Verification items for the finished model (mm, model axes). A direction names the side the tool comes from. Round coordinates to 2 decimals unless told otherwise and drop trailing zeros. Loops run counter-clockwise (first coordinate to the right, second up) from the corner with the lowest first, then second, coordinate; pieces in that order, holes last.
from build123d import *

# Parameters (mm, degrees)
EXTRUDE_1_DEPTH     = 90
CUT_EXTRUDE_1_DEPTH = 160
SKETCH_4_W          = 100
SKETCH_4_H          = 40
CUT_EXTRUDE_2_DEPTH = 102.056914657
SKETCH_5_R          = 5
CUT_EXTRUDE_3_DEPTH = 102.056914657
SKETCH_6_R          = 2.5
CUT_EXTRUDE_4_DEPTH = 102.056914657


with BuildPart() as part:
    # 草圖1 → 填料-伸長1 (new, symmetric)
    with BuildSketch(Plane(origin=(0, 0, 0), x_dir=(0, 0, -1), z_dir=(1, 0, 0))):
        Polygon((-59.343145751, 0), (-13.343145751, 46), (0, 46), (0, 50), (-15, 50), (-62.171572875, 2.828427125), align=None)
    extrude(amount=EXTRUDE_1_DEPTH, both=True)

    # 草圖3 → 除料-伸長1 (cut)
    with BuildSketch(Plane(origin=(0, 0, 0), x_dir=(1, 0, 0), z_dir=(0, 1, 0))):
        Polygon((-90, -15), (-90, -62.171572875), (-80, -62.171572875), align=None)
        Polygon((90, -15), (80, -62.171572875), (90, -62.171572875), align=None)
    extrude(amount=CUT_EXTRUDE_1_DEPTH, mode=Mode.SUBTRACT)

    # 草圖4 → 除料-伸長2 (cut, through all)
    with BuildSketch(Plane(origin=(0, 32.5, 32.5), x_dir=(1, 0, 0), z_dir=(0, 0.7071067811865467, 0.7071067811865485))):
        with Locations((-15, -11.961940777)):
            Rectangle(SKETCH_4_W, SKETCH_4_H)
    extrude(amount=-CUT_EXTRUDE_2_DEPTH, mode=Mode.SUBTRACT)

    # 草圖5 → 除料-伸長3 (cut, through all)
    with BuildSketch(Plane(origin=(0, 32.5, 32.5), x_dir=(1, 0, 0), z_dir=(0, 0.7071067811865467, 0.7071067811865485))):
        with Locations(Location((60, -11.961940777, 0), (0, 0, 270))):
            Circle(SKETCH_5_R)
    extrude(amount=-CUT_EXTRUDE_3_DEPTH, mode=Mode.SUBTRACT)

    # 草圖6 → 除料-伸長4 (cut, through all)
    with BuildSketch(Plane(origin=(0, 32.5, 32.5), x_dir=(1, 0, 0), z_dir=(0, 0.7071067811865467, 0.7071067811865485))):
        with Locations(Location((70, -31.961940777, 0), (0, 0, 270))):
            Circle(SKETCH_6_R)
        with Locations(Location((70, 18.038059223, 0), (0, 0, 270))):
            Circle(SKETCH_6_R)
    cut_extrude_4 = extrude(amount=-CUT_EXTRUDE_4_DEPTH, mode=Mode.SUBTRACT)

    # 鏡射1: 除料-伸長4 across plane
    add(cut_extrude_4.mirror(Plane(origin=(0, 0, 0), x_dir=(0, 0, 1), z_dir=(1, 0, 0))), mode=Mode.SUBTRACT)


solid = part.part
1. Section check A-A (x = -27). Enter the section's corners in (y, z), then the cut area to 3 significant figures.
2. Gauge pin test, flat ends, axial feed: P1, Ø15.5, axis at y = 25.5, z = 34, coming from the +X side; P2, Ø3, axis at y = 42, z = 22, coming from the -X side; P3, Ø6.5, axis at x = 5.5, z = 5, coming from the -Y side. Record the tip position at first contact, or that the pin passes through.
3. Section check D-D (x = 40). Enter the section's corners in (y, z).
4. Section check B-B (y = 14.5). Enter the section's corners in (x, z).
5. Release check for a two-part mould opening along X. For faces 1 (the face through (-84.977, 24.883, 38.696)), 2 (the face through (67.56, 44.24, 17.97)), 3 (the face through (1, 50, 7)), 4 (the face through (85.023, 24.883, 38.476)) record: released by +X, released by -X, zero draft, split by the parting line, or undercut.
6. Scan lines: L1, parallel to X at y = 9, z = 53; L2, parallel to Y at x = -61.5, z = 12; L3, parallel to X at y = 3, z = 59.5. Record each from-to range of solid material in increasing order.
7. Section check C-C (z = 48). Enter the section's corners in (x, y), then the cut area to 3 significant figures.
8. Tool access check on faces 5 (the face through (1, 48, 0)), 6 (the face through (1, 46, 7)). Record the directions out of +Z, -Z, +X, -X, +Y, -Y that give a thin tool (end or side, any length) a straight path to the whole face; none if there is none.
Taken from the geometry:
1. outline: (0, 59.34) - (7.07, 52.27) - (9.9, 55.1) - (2.83, 62.17) - close; (35.36, 23.99) - (46, 13.34) - (46, 0) - (50, 0) - (50, 15) - (38.18, 26.82) - close
1. area: 160 mm2
2. P1: stops at x = 87.15
2. P2: stops at x = -88.83
2. P3: stops at y = 46
3. outline: (0, 59.34) - (46, 13.34) - (46, 0) - (50, 0) - (50, 15) - (2.83, 62.17) - close
4. outline: (-83.67, 44.84) - (-65, 44.84) - (-65, 50.5) - (-82.47, 50.5) - close; (35, 44.84) - (83.67, 44.84) - (82.47, 50.5) - (35, 50.5) - close
5. face 1: released by -X
5. face 2: undercut
5. face 3: zero draft
5. face 4: released by +X
6. L1: x = -81.94 to -72.35, -67.65 to -65, 35 to 67.65, 72.35 to 81.94
6. L2: y = 46 to 50
6. L3: x = -80.57 to 80.57
7. outline: (-83, 11.34) - (-65, 11.34) - (-65, 17) - (-83, 17) - close; (35, 11.34) - (83, 11.34) - (83, 17) - (35, 17) - close
7. area: 373 mm2
8. face 5: -Z, +X, -X, +Y, -Y
8. face 6: -Z, +X, -X, -Y
